Geometry: final body of the model. Coordinates: model frame, mm. Face numbers are marked on the shaded views. Give positions to 0.01 mm unless a question says otherwise; leave off trailing zeros. Loops run counter-clockwise (first coordinate to the right, second up) from the corner with the lowest first, then second, coordinate; pieces in that order, holes last. Notation, with made-up numbers: (46, 82) - (96, 82) arc R36 ccw to (96, 117) - close; hole circle Ø6 at (53.5, -35.5). An arc over 180 degrees is marked (long way). Use one line per item in the form item = value.
```python
from build123d import *

# Parameters (mm, degrees)
F1_DEPTH      = 680
F3_D          = 5
F4_R          = 2
F6_DEPTH      = 25
F6_DEPTH_BACK = 25


# Not quite as in the source:
# - a feature names something its author has since deleted; it is built from what else it names


with BuildPart() as f1:
    # F0 (on Right) → F1 (new body)
    with BuildSketch(Plane.YZ):
        Polygon((-18.8378913403, 177.8021101952), (-18.8378913403, 154.8021101952), (-16.8378913403, 154.8021101952), (-16.8378913403, 179.8021101952), (-56.8378913403, 179.8021101952), (-56.8378913403, 79.8021101952), (-29.8378913403, 79.8021101952), (-29.8378913403, 53.8021101952), (-27.8378913403, 53.8021101952), (-27.8378913403, 81.8021101952), (-54.8378913403, 81.8021101952), (-54.8378913403, 177.8021101952), align=None)
    extrude(amount=F1_DEPTH)

    # F3 (through all)
    with Locations(Plane.XZ.offset(29.8378913403)):
        with Locations((580, 66.8021101952), (100, 66.8021101952)):
            Hole(F3_D / 2)

    # F4
    f4_edges = [f1.edges().sort_by_distance(p)[0] for p in [
        (340, -56.837891, 179.80211),
        (340, -16.837891, 179.80211),
        (340, -56.837891, 79.80211),
        (340, -27.837891, 81.80211),
        (340, -54.837891, 81.80211),
        (340, -29.837891, 79.80211),
        (340, -18.837891, 177.80211),
        (340, -54.837891, 177.80211),
    ]]
    fillet(f4_edges, radius=F4_R)

    # F5 (on face) → F6 (join, two sides)
    with BuildSketch(Plane.YZ.offset(680)) as f6_sk:
        with BuildLine():
            Line((-20.8378913403, 154.8021101952), (-18.8378913403, 154.8021101952))
            Line((-18.8378913403, 154.8021101952), (-18.8378913403, 175.8021101952))
            ThreePointArc((-18.8378913403, 175.8021101952), (-19.4236777779, 177.2163237575), (-20.8378913403, 177.8021101952))
            Line((-20.8378913403, 177.8021101952), (-52.8378913403, 177.8021101952))
            ThreePointArc((-52.8378913403, 177.8021101952), (-54.2521049026, 177.2163237575), (-54.8378913403, 175.8021101952))
            Line((-54.8378913403, 175.8021101952), (-54.8378913403, 83.8021101952))
            ThreePointArc((-54.8378913403, 83.8021101952), (-54.2521049026, 82.3878966328), (-52.8378913403, 81.8021101952))
            Line((-52.8378913403, 81.8021101952), (-29.8378913403, 81.8021101952))
            Line((-29.8378913403, 81.8021101952), (-29.8378913403, 83.8021101952))
            Line((-29.8378913403, 83.8021101952), (-52.8378913403, 83.8021101952))
            Line((-52.8378913403, 83.8021101952), (-52.8378913403, 175.8021101952))
            Line((-52.8378913403, 175.8021101952), (-20.8378913403, 175.8021101952))
            Line((-20.8378913403, 175.8021101952), (-20.8378913403, 154.8021101952))
        make_face()
    extrude(amount=F6_DEPTH)
    extrude(f6_sk.sketch, amount=-F6_DEPTH_BACK)


solid = f1.part
```
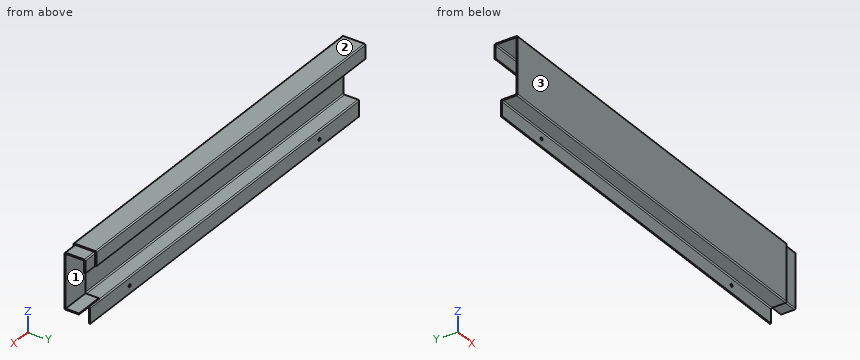
(1) Material intervals for L1, parallel to Z at x = 580, y = -28.95; L2, parallel to Y at x = 517.5, z = 160; L3, parallel to Z at x = 554, y = -37, sorted ascending. Write a range as from..to.
Solution:
L1 = 53.8..64.3, 69.3..81.59, 177.8..179.8
L2 = -56.84..-54.84, -18.84..-16.84
L3 = 79.8..81.8, 177.8..179.8
(2) Pin query (flat end, axial travel): P1, Ø2, axis at y = -50.5, z = 114.5, coming from the +X side; P2, Ø9.5, axis at x = 683.5, y = -35, coming from the -Z side; P3, Ø25, axis at x = 672, z = 126.5, coming from the +Y side; P4, Ø17, axis at x = 693.5, z = 164, coming from the +Y side. Return the tip coordinate at first contact, or that it passes through.
Solution:
P1 = through
P2 = 79.8
P3 = -52.84
P4 = -18.84
(3) Pull-direction query (Z, two-part tool) for the marked faces 1, 2 and 3; classes: released by +Z, released by -Z, zero draft, split by the parting line, or undercut.
Solution:
face_1 = undercut
face_2 = released by +Z
face_3 = zero draft
(4) Cut plane C-C (x = 459). Return the cut outline in (y, z).
Solution:
outline = (-56.84, 81.8) arc R2 ccw to (-54.84, 79.8) - (-31.84, 79.8) arc R2 cw to (-29.84, 77.8) - (-29.84, 53.8) - (-27.84, 53.8) - (-27.84, 79.8) arc R2 ccw to (-29.84, 81.8) - (-52.84, 81.8) arc R2 cw to (-54.84, 83.8) - (-54.84, 175.8) arc R2 cw to (-52.84, 177.8) - (-20.84, 177.8) arc R2 cw to (-18.84, 175.8) - (-18.84, 154.8) - (-16.84, 154.8) - (-16.84, 177.8) arc R2 ccw to (-18.84, 179.8) - (-54.84, 179.8) arc R2 ccw to (-56.84, 177.8) - close
(5) Cut plane A-A (y = -46.5). Return the cut outline in (x, z), plus the area to 3 significant figures.
Solution:
outline = (0, 79.8) - (680, 79.8) - (680, 81.8) - (705, 81.8) - (705, 83.8) - (655, 83.8) - (655, 81.8) - (0, 81.8) - close; (0, 177.8) - (655, 177.8) - (655, 175.8) - (705, 175.8) - (705, 177.8) - (680, 177.8) - (680, 179.8) - (0, 179.8) - close
area = 2,920 mm2
(6) Cut plane B-B (z = 137). Return the cut outline in (x, y).
Solution:
outline = (0, -56.84) - (680, -56.84) - (680, -54.84) - (705, -54.84) - (705, -52.84) - (655, -52.84) - (655, -54.84) - (0, -54.84) - close
